Design review of the part built by this model. Coordinates are the model's own, in mm. A direction names the side the tool comes from. Coordinates: 2 decimals unless noted, no trailing zeros. Order: outer loops, then holes, each group sorted by start corner. A loop starts at its lowest first (then second) coordinate and runs counter-clockwise, first axis right, second up. Notation, with made-up numbers: M 19,32.25 L 47,32.25 A21 ccw 47,57.25 Z; hole C 5.25,84.25 d10. An arc over 180 degrees is marked long. Answer as a JSON object with one key per item and string values.
from build123d import *

# Parameters (mm, degrees)
F0_R     = 2.15
F1_DEPTH = 3


with BuildPart() as f1:
    # F0 (on Top) → F1 (new body)
    with BuildSketch(Plane.XY):
        with BuildLine():
            ThreePointArc((15, 35), (13.535534, 38.535534), (10, 40))
            Line((10, 40), (-10, 40))
            ThreePointArc((-10, 40), (-13.535534, 38.535534), (-15, 35))
            Line((-15, 35), (-15, -35))
            ThreePointArc((-15, -35), (-13.535534, -38.535534), (-10, -40))
            Line((-10, -40), (10, -40))
            ThreePointArc((10, -40), (13.535534, -38.535534), (15, -35))
            Line((15, -35), (15, 35))
        make_face()
        with Locations((-7.5, -30)):
            Circle(F0_R, mode=Mode.SUBTRACT)
        with Locations((7.5, -15)):
            Circle(F0_R, mode=Mode.SUBTRACT)
        with BuildLine():
            Line((5.5, 12), (-5.5, 12))
            ThreePointArc((-5.5, 12), (-6.353553, 11.646447), (-6, 12.5))
            Line((-6, 12.5), (-6, 14.5))
            ThreePointArc((-6, 14.5), (-6.353553, 15.353553), (-5.5, 15))
            Line((-5.5, 15), (5.5, 15))
            ThreePointArc((5.5, 15), (6, 15.5), (6.5, 15))
            ThreePointArc((6.5, 15), (6.353553, 14.646447), (6, 14.5))
            Line((6, 14.5), (6, 12.5))
            ThreePointArc((6, 12.5), (6.353553, 12.353553), (6.5, 12))
            ThreePointArc((6.5, 12), (6, 11.5), (5.5, 12))
        make_face(mode=Mode.SUBTRACT)
        with BuildLine():
            Line((5.5, 25), (-5.5, 25))
            ThreePointArc((-5.5, 25), (-6.353553, 24.646447), (-6, 25.5))
            Line((-6, 25.5), (-6, 27.5))
            ThreePointArc((-6, 27.5), (-6.353553, 28.353553), (-5.5, 28))
            Line((-5.5, 28), (5.5, 28))
            ThreePointArc((5.5, 28), (6, 28.5), (6.5, 28))
            ThreePointArc((6.5, 28), (6.353553, 27.646447), (6, 27.5))
            Line((6, 27.5), (6, 25.5))
            ThreePointArc((6, 25.5), (6.353553, 25.353553), (6.5, 25))
            ThreePointArc((6.5, 25), (6, 24.5), (5.5, 25))
        make_face(mode=Mode.SUBTRACT)
    extrude(amount=F1_DEPTH)


solid = f1.part
1) Add section C-C (x = -7.5). State the section outline as (y, z) points.
Taken from the geometry:
{"outline": "M -40,0 L -32.15,0 L -32.15,3 L -40,3 Z; M -27.85,0 L 40,0 L 40,3 L -27.85,3 Z"}
2) Add section B-B (z = 0.55). Count the separate pieces of the cut face and the enclosed holes in it, and give its area (3 significant figures).
Taken from the geometry:
{"separate pieces": "1", "enclosed holes": "4", "area": "2,270 mm2"}
3) Tool access review of faces 1 (the flat face through (0, 1, 0)), 2 (the flat face through (-6, 26, 1)): name each direction out of +Z, -Z, +X, -X, +Y, -Y from which nothing blocks a thin tool from reaching the whole face with its end or side.
Taken from the geometry:
{"face 1": "-Z, +X, -X, +Y, -Y", "face 2": "+Z, -Z"}
4) Insertion check: pin 1 Ø10 at (x, y) = (-9, 18.5) entering from -Z; pin 2 Ø2.5 at (x, y) = (7.5, -15) entering from -Z. Each pin has a flat end and moves straight along its axis. Give the tip position at first contact, or say it passes through.
Taken from the geometry:
{"pin 1": "stops at z = 0", "pin 2": "passes through"}
5) To check wall thickness, follow L1, parallel to Y at x = 0.5, z = 2.8; L2, parallel to Y at x = 7.5, z = 1.55; L3, parallel to Y at x = 11.5, z = 0.45. State the ranges of each line that lie inside material, in increasing order.
Taken from the geometry:
{"L1": "y = -40 to 12, 15 to 25, 28 to 40", "L2": "y = -40 to -17.15, -12.85 to 40", "L3": "y = -39.77 to 39.77"}
6) Add section A-A (x = -1). State the section outline as (y, z) points, and give its area (3 significant figures).
Taken from the geometry:
{"outline": "M -40,0 L 12,0 L 12,3 L -40,3 Z; M 15,0 L 25,0 L 25,3 L 15,3 Z; M 28,0 L 40,0 L 40,3 L 28,3 Z", "area": "222 mm2"}
7) Add section D-D (y = -30). State the section outline as (x, z) points, and give its area (3 significant figures).
Taken from the geometry:
{"outline": "M -15,0 L -9.65,0 L -9.65,3 L -15,3 Z; M -5.35,0 L 15,0 L 15,3 L -5.35,3 Z", "area": "77.1 mm2"}
